The listing builds one solid part. Answer for the finished solid, in the listing's coordinates (mm). A direction names the side the tool comes from. Coordinates: 2 decimals unless noted, no trailing zeros. Loops run counter-clockwise (first coordinate to the right, second up) from the corner with the lowest first, then second, coordinate; pieces in that order, holes last. Notation, with made-up numbers: (65, -27) - (113, -27) arc R13 ccw to (113, -7) - close; hole circle Ø3 at (13.25, -28). An arc over 180 degrees is marked (long way). One line per question, with ' | ' between items.
from build123d import *
from build123d.topology import SkipClean

# Parameters (mm, degrees)
SKETCH_1_R          = 2.6
EXTRUDE_1_DEPTH     = 4.5
EXTRUDE_START       = 4.5
SKETCH_2_R          = 12.9
EXTRUDE_2_DEPTH     = 3
EXTRUDE_START_2     = 7.5
SKETCH_4_R          = 6.1
EXTRUDE_3_DEPTH     = 3
SKETCH_6_R          = 4
CUT_EXTRUDE_1_DEPTH = 10.5


with BuildPart() as part:
    # 草图1 → 凸台-拉伸1 (new body)
    with BuildSketch(Plane.XY):
        with BuildLine():
            Line((-20.635135135, 4.521194306), (-5.508648649, 11.66468131))
            ThreePointArc((-5.508648649, 11.66468131), (0, 12.9), (5.508648649, 11.66468131))
            Line((5.508648649, 11.66468131), (20.635135135, 4.521194306))
            ThreePointArc((20.635135135, 4.521194306), (23.5, 0), (20.635135135, -4.521194306))
            Line((20.635135135, -4.521194306), (5.508648649, -11.66468131))
            ThreePointArc((5.508648649, -11.66468131), (0, -12.9), (-5.508648649, -11.66468131))
            Line((-5.508648649, -11.66468131), (-20.635135135, -4.521194306))
            ThreePointArc((-20.635135135, -4.521194306), (-23.5, 0), (-20.635135135, 4.521194306))
        make_face()
        with Locations((18.5, 0)):
            Circle(SKETCH_1_R, mode=Mode.SUBTRACT)
        with Locations((-18.5, 0)):
            Circle(SKETCH_1_R, mode=Mode.SUBTRACT)
    extrude(amount=EXTRUDE_1_DEPTH)

    # 草图2 → 凸台-拉伸2 (add)
    with SkipClean():  # the faces are left unmerged after this step: merging them gives an invalid solid
        with BuildSketch(Plane.XY.offset(EXTRUDE_START)):
            with Locations(Location((0, 0, 0), (0, 0, 115.279035224))):
                Circle(SKETCH_2_R)
        extrude(amount=EXTRUDE_2_DEPTH)

    # 草图4 → 凸台-拉伸3 (add)
    with SkipClean():  # the faces are left unmerged after this step: merging them gives an invalid solid
        with BuildSketch(Plane.XY.offset(EXTRUDE_START_2)):
            Circle(SKETCH_4_R)
        extrude(amount=EXTRUDE_3_DEPTH)

    # 草图6 → 切除-拉伸1 (cut)
    with SkipClean():  # the faces are left unmerged after this step: merging them gives an invalid solid
        with BuildSketch(Plane.XY):
            Circle(SKETCH_6_R)
        extrude(amount=CUT_EXTRUDE_1_DEPTH, mode=Mode.SUBTRACT)


solid = part.part
Item 1: Each of these flat-tipped pins is pushed along its axis until it touches: pin 1 Ø5.5 at (x, y) = (11.5, 6) entering from +Z; pin 2 Ø4.5 at (x, y) = (18.5, 0) entering from -Z; pin 3 Ø2 at (y, z) = (-5.5, 3.5) entering from +X; pin 4 Ø5 at (y, z) = (3.5, 4.5) entering from +X. Where does it stop, or does it pass through?
Taken from the geometry:
pin 1: stops at z = 7.5 | pin 2: passes through | pin 3: stops at x = 20.68 | pin 4: stops at x = 23.4
Item 2: Find section A-A, the plane y = 0. Write down the section's boundary in (x, z), plus the area to 3 significant figures.
Taken from the geometry:
outline: (-23.5, 0) - (-21.1, 0) - (-21.1, 4.5) - (-23.5, 4.5) - close; (-15.9, 0) - (-4, 0) - (-4, 10.5) - (-6.1, 10.5) - (-6.1, 7.5) - (-12.9, 7.5) - (-12.9, 4.5) - (-15.9, 4.5) - close; (4, 0) - (15.9, 0) - (15.9, 4.5) - (12.9, 4.5) - (12.9, 7.5) - (6.1, 7.5) - (6.1, 10.5) - (4, 10.5) - close; (21.1, 0) - (23.5, 0) - (23.5, 4.5) - (21.1, 4.5) - close | area: 195 mm2
Item 3: Find the intervals of material crossed by line 1 (Z direction, x = -6.5, y = 8.5); line 2 (Y direction, x = -3.5, z = 4.25); line 3 (Y direction, x = 0, z = 4.75), in increasing order. Write a range as [from, to].
Taken from the geometry:
line 1: z = [0, 7.5] | line 2: y = [-12.42, -1.94], [1.94, 12.42] | line 3: y = [-12.9, -4], [4, 12.9]
Item 4: Find section C-C, the plane z = 1.5. Write down the section's boundary in (x, y).
Taken from the geometry:
outline: (-20.64, -4.52) - (-5.51, -11.66) arc R12.9 ccw to (5.51, -11.66) - (20.64, -4.52) arc R5 ccw to (20.64, 4.52) - (5.51, 11.66) arc R12.9 ccw to (-5.51, 11.66) - (-20.64, 4.52) arc R5 ccw to start; hole circle Ø5.2 at (-18.5, 0); hole circle Ø8 at (0, 0); hole circle Ø5.2 at (18.5, 0)
Item 5: The mould has two halves that part along Y. Classify faces 1 (the face through (4, -1.3, 10.5)), 2 (the face through (20.98, 0.78, 2.22)), 3 (the face through (-16.02, 0.78, 2.22)), 4 (the face through (-6.094, 0.268, 8.979)): pulls with the +Y half, pulls with the -Y half, needs draft (parallel to the pull), parting line crosses it, or undercut.
Taken from the geometry:
face 1: needs draft | face 2: undercut | face 3: undercut | face 4: parting line crosses it
Item 6: Find section B-B, the plane x = 0. Write down the section's boundary in (y, z).
Taken from the geometry:
outline: (-12.9, 0) - (-4, 0) - (-4, 10.5) - (-6.1, 10.5) - (-6.1, 7.5) - (-12.9, 7.5) - close; (4, 0) - (12.9, 0) - (12.9, 7.5) - (6.1, 7.5) - (6.1, 10.5) - (4, 10.5) - close
Item 7: Which of the six approach directions +Z, -Z, +X, -X, +Y, -Y give full straight-line access (tool end or side, diameter ignored) to faces 5 (the face through (-12.97, -8.14, 2.22)), 6 (the face through (4, 5, 7.5))?
Taken from the geometry:
face 5: +Z, -Z, -X, -Y | face 6: +Z
Item 8: Find section D-D, the plane z = 5. Write down the section's boundary in (x, y), plus the area to 3 significant figures.
Taken from the geometry:
outline: circle Ø25.8 at (0, 0); hole circle Ø8 at (0, 0) | area: 473 mm2
